```python
from build123d import *

# Parameters (mm, degrees)
F1_DEPTH = 25.4
F3_DEPTH = 25.4
F4_DEPTH = 25.4
F5_D     = 6.35
F6_D     = 6.35
F7_D     = 6.35


with BuildPart() as f1:
    # F0 (on Front) → F1 (new body)
    with BuildSketch(Plane.XZ):
        with BuildLine():
            ThreePointArc((-81.4044819336, 83.7894535693), (-56.9535815274, 83.462929282), (-44.8214243022, 62.2317279536))
            ThreePointArc((-44.8214243022, 62.2317279536), (-67.8461689377, 37.641623994), (-93.8954395614, 59.0015766684))
            Line((-93.8954395614, 59.0015766684), (-85.9510365488, -1.0845648523))
            ThreePointArc((-85.9510365488, -1.0845648523), (-63.3331540861, 26.4987987528), (-37.294890351, 2.1180814432))
            ThreePointArc((-37.294890351, 2.1180814432), (-38.734729228, -6.1455375994), (-42.8845494933, -13.4352239739))
            Line((-42.8845494933, -13.4352239739), (-7.1169419868, 29.8995050449))
            Line((-7.1169419868, 29.8995050449), (37.9090425379, -0.3676435997))
            ThreePointArc((37.9090425379, -0.3676435997), (38.1002397013, 23.7171988773), (60.1805807204, 14.0956223965))
            Line((60.1805807205, 14.0956223965), (45.3402720787, 99.0440562508))
            ThreePointArc((45.3402720787, 99.0440562508), (45.7257653294, 96.0179672104), (45.8545692558, 92.9701434826))
            ThreePointArc((45.8545692558, 92.9701434826), (-8.6091784666, 61.8478937228), (-7.7715557558, 124.5710364556))
            Line((-7.7715557558, 124.5710364556), (-81.4044819336, 83.7894535693))
        make_face()
        with BuildLine():
            Line((-4.2810993854, 33.3353085342), (-7.1169419868, 29.8995050449))
            Line((-7.1169419868, 29.8995050449), (-10.8142049734, 32.3848612137))
            ThreePointArc((-10.8142049734, 32.3848612137), (-10.3830468788, 40.8024385377), (-3.1566041276, 36.4642326329))
            ThreePointArc((-3.1566041276, 36.4642326329), (-3.4462625741, 34.8018055217), (-4.2810993854, 33.3353085342))
        make_face(mode=Mode.SUBTRACT)
        with BuildLine():
            ThreePointArc((45.2904246952, 99.3293910955), (25.2484905686, 125.5912487777), (-7.7715557558, 124.5710364556))
            ThreePointArc((-7.7715557558, 124.5710364556), (-8.6091784666, 61.8478937228), (45.8545692558, 92.9701434826))
            ThreePointArc((45.8545692558, 92.9701434826), (45.7257653294, 96.0179672104), (45.3402720787, 99.0440562508))
            Line((45.3402720787, 99.0440562508), (45.2904246952, 99.3293910955))
        make_face()
        with BuildLine():
            ThreePointArc((-93.8954395614, 59.0015766684), (-67.8461689377, 37.641623994), (-44.8214243022, 62.2317279536))
            ThreePointArc((-44.8214243022, 62.2317279536), (-56.9535815274, 83.462929282), (-81.4044819336, 83.7894535693))
            ThreePointArc((-81.4044819336, 83.7894535693), (-91.4718288588, 73.321407878), (-93.8954395614, 59.0015766684))
        make_face()
        with BuildLine():
            ThreePointArc((-37.294890351, 2.1180814432), (-63.3331540861, 26.4987987528), (-85.9510365488, -1.0845648523))
            ThreePointArc((-85.9510365488, -1.0845648523), (-68.4639217442, -21.3686596672), (-42.8845494933, -13.4352239739))
            ThreePointArc((-42.8845494933, -13.4352239739), (-38.734729228, -6.1455375994), (-37.294890351, 2.1180814432))
        make_face()
        with BuildLine():
            ThreePointArc((60.3959257616, 11.6116108139), (60.3419887269, 12.858275066), (60.1805807204, 14.0956223965))
            ThreePointArc((60.1805807204, 14.0956223965), (38.1002397013, 23.7171988773), (37.9090425379, -0.3676435997))
            ThreePointArc((37.9090425379, -0.3676435997), (52.7482001902, -1.1277225028), (60.3959257616, 11.6116108139))
        make_face()
        with BuildLine():
            Line((-10.8142049734, 32.3848612137), (-7.1169419868, 29.8995050449))
            Line((-7.1169419868, 29.8995050449), (-4.2810993854, 33.3353085342))
            ThreePointArc((-4.2810993854, 33.3353085342), (-7.3643405271, 31.6000525145), (-10.8142049734, 32.3848612137))
        make_face()
        with BuildLine():
            ThreePointArc((45.3402720787, 99.0440562508), (45.315634379, 99.1867736354), (45.2904246952, 99.3293910955))
            Line((45.2904246952, 99.3293910955), (45.3402720787, 99.0440562508))
        make_face()
    extrude(amount=F1_DEPTH)

    # F2 (on face) → F3 (cut)
    with BuildSketch(Plane.XZ.offset(25.4)):
        Polygon((-52.0894788206, 47.2524687648), (-35.853933543, 66.2599354982), (-60.4326552345, 70.8165967862), align=None)
    extrude(amount=-F3_DEPTH, mode=Mode.SUBTRACT)

    # F2 (on face) → F4 (cut)
    with BuildSketch(Plane.XZ.offset(25.4)):
        Polygon((-27.510757129, 42.6958074768), (-35.853933543, 66.2599354982), (-52.0894788206, 47.2524687648), align=None)
    extrude(amount=-F4_DEPTH, mode=Mode.SUBTRACT)

    # F5 (through all)
    with Locations(Plane.XZ.offset(25.4)):
        with Locations((-19.6183882654, 85.2674022317)):
            Hole(F5_D / 2)

    # F6 (through all)
    with Locations(Plane.XZ.offset(25.4)):
        with Locations((-44.1971099569, 89.8240635197)):
            Hole(F6_D / 2)

    # F7 (through all)
    with Locations(Plane.XZ.offset(25.4)):
        with Locations((-11.2752118514, 61.7032742103)):
            Hole(F7_D / 2)


solid = f1.part
```
Model file for the job. Use its own axes, mm. A direction names the side the tool comes from. Coordinates: 2 decimals unless noted, no trailing zeros. Loops run counter-clockwise (first coordinate to the right, second up) from the corner with the lowest first, then second, coordinate; pieces in that order, holes last. Notation, with made-up numbers: (-13, 70) -> (24, 70) arc R34 cw to (24, 109) -> close; hole circle Ø10 at (4, 51). An arc over 180 degrees is marked (long way). Answer as a JSON object with one key per item and string values.
Q1. Flat gauge pins, fed straight in: P1, Ø4, axis at y = -11.5, z = 69.5, coming from the +X side; P2, Ø12, axis at y = -17.5, z = 49.5, coming from the +X side; P3, Ø6, axis at x = -50.5, y = -13.5, coming from the -Z side. Where does each tip first touch, or does it go through?
Report:
{"P1": "stops at x = 50.85", "P2": "stops at x = 55.04", "P3": "stops at z = -20.89"}
Q2. Probe probe 1 along X at (y, z) = (-10.75, 19.5); probe 2 along X at (y, z) = (-11.5, 4); probe 3 along Z at (x, y) = (-43.5, -13.25). List the from-to ranges inside material, lowest first.
Report:
{"probe 1": "x = -88.67 to -15.7, 8.35 to 59.24", "probe 2": "x = -86.62 to -28.49, 31.41 to 58.23", "probe 3": "z = -14.15 to 45.66, 67.68 to 86.73, 92.92 to 104.78"}
Q3. Cut at C-C (x = 26). List the corners of the cut face in (y, z).
Report:
{"outline": "(-25.4, 7.64) -> (0, 7.64) -> (0, 125.22) -> (-25.4, 125.22) -> close"}
Q4. Cut at A-A (y = -19.5). State how many separate pieces and enclosed holes the cut face has, and give its area (3 significant figures).
Report:
{"separate pieces": "1", "enclosed holes": "5", "area": "15,000 mm2"}
Q5. Pull direction X, two halves, no side cores. Call faces 1 (the flat face through (52.864, -12.522, 55.975)), 2 (the cylindrical face through (-68.844, -12.522, -21.256)), 3 (the flat face through (-39.972, -12.878, 45.006)), 4 (the cylindrical face through (-10.6, -12.5, 58.6)): released by +X, released by -X, zero draft, split by the parting line, or undercut.
Report:
{"face 1": "released by +X", "face 2": "split by the parting line", "face 3": "undercut", "face 4": "undercut"}
Q6. Cut at D-D (z = 3). List the corners of the cut face in (x, y).
Report:
{"outline": "(-86.49, -25.4) -> (-29.32, -25.4) -> (-29.32, 0) -> (-86.49, 0) -> close; (32.9, -25.4) -> (57.55, -25.4) -> (57.55, 0) -> (32.9, 0) -> close"}
Q7. Cut at B-B (z = 54). List the corners of the cut face in (x, y).
Report:
{"outline": "(-93.23, -25.4) -> (-54.48, -25.4) -> (-54.48, 0) -> (-93.23, 0) -> close; (-31.51, -25.4) -> (53.21, -25.4) -> (53.21, 0) -> (-31.51, 0) -> close"}
Q8. 3-axis set-ups, long thin cutter, end or side, ignore diameter. For faces 5 (the flat face through (-25.25, -12.52, 7.93)), 6 (the flat face through (-47.971, -12.878, 68.506)), 7 (the flat face through (-18, -25.4, 54)): which of +Z, -Z, +X, -X, +Y, -Y reach the whole face in a straight line?
Report:
{"face 5": "-Z, +Y, -Y", "face 6": "+Y, -Y", "face 7": "+Z, -Z, +X, -X, -Y"}
